Source: CAD feature listing. Evaluate the final solid. Frame: model axes, mm. Face numbers are marked on the shaded views. A direction names the side the tool comes from. Give positions to 0.01 mm unless a question says otherwise; leave off trailing zeros. Write each loop counter-clockwise with the first axis right and the second up, starting at its lowest first coordinate (ties: lowest second). Pieces come first, ordered by that corner, then holes. Notation, with made-up numbers: (38, -22.75) -> (95, -22.75) arc R32 ccw to (95, 15.25) -> close; hole circle Ø10 at (-31.5, -31.5). An arc over 180 degrees is marked (long way). Use a Markdown table: item, result. Add a question column.
```python
from build123d import *

# Parameters (mm, degrees)
SKETCH1_W           = 120
SKETCH1_H           = 25
BOSS_EXTRUDE4_DEPTH = 1
SKETCH6_W           = 76
SKETCH6_H           = 7.5
CUT_EXTRUDE1_DEPTH  = 62.296410988
SKETCH7_W           = 1
SKETCH7_H           = 25
BOSS_EXTRUDE5_DEPTH = 23
SKETCH11_R          = 1.5
SKETCH11_W          = 6
SKETCH11_H          = 12
CUT_EXTRUDE3_DEPTH  = 66.819829839
CUT_EXTRUDE4_DEPTH  = 1
CUT_EXTRUDE5_DEPTH  = 1
BOSS_EXTRUDE6_DEPTH = 1
SKETCH13_W          = 22
SKETCH13_H          = 1
BOSS_EXTRUDE7_DEPTH = 1
SKETCH16_R          = 1.5
CUT_EXTRUDE6_DEPTH  = 1
SKETCH17_R          = 1.5
CUT_EXTRUDE7_DEPTH  = 1
CUT_EXTRUDE8_REACH  = 69.218


with BuildPart() as part:
    # Sketch1 → Boss-Extrude4 (new body)
    with BuildSketch(Plane.XY):
        Rectangle(SKETCH1_W, SKETCH1_H)
    extrude(amount=BOSS_EXTRUDE4_DEPTH)

    # Sketch6 → Cut-Extrude1 (cut, through all)
    with BuildSketch(Plane(origin=(0, 0, 0), x_dir=(-1, 0, 0), z_dir=(0, 0, -1))):
        with Locations((0, 8.75)):
            Rectangle(SKETCH6_W, SKETCH6_H)
        with Locations((0, -8.75)):
            Rectangle(SKETCH6_W, SKETCH6_H)
    extrude(amount=-CUT_EXTRUDE1_DEPTH, mode=Mode.SUBTRACT)

    # Sketch7 → Boss-Extrude5 (add)
    with BuildSketch(Plane.XY.offset(1)):
        with Locations((-38.5, 0)):
            Rectangle(SKETCH7_W, SKETCH7_H)
    extrude(amount=BOSS_EXTRUDE5_DEPTH)

    # Sketch11 → Cut-Extrude3 (cut, through all)
    with BuildSketch(Plane(origin=(0, 0, 0), x_dir=(-1, 0, 0), z_dir=(0, 0, -1))):
        with Locations((-49, 10)):
            Circle(SKETCH11_R)
        with Locations((-49, -10)):
            Circle(SKETCH11_R)
        with Locations((-49, 0)):
            Rectangle(SKETCH11_W, SKETCH11_H)
    extrude(amount=-CUT_EXTRUDE3_DEPTH, mode=Mode.SUBTRACT)

    # Sketch14 → Cut-Extrude4 (cut)
    with BuildSketch(Plane(origin=(0, 12.5, 0), x_dir=(1, 0, 0), z_dir=(0, 1, 0))):
        Polygon((-60, -1), (-39, -1), (-39, -24), (-38, -24), (-38, 0), (-60, 0), align=None)
    extrude(amount=-CUT_EXTRUDE4_DEPTH, mode=Mode.SUBTRACT)

    # Sketch15 → Cut-Extrude5 (cut)
    with BuildSketch(Plane.XZ.offset(12.5)):
        Polygon((-60, 0), (-38, 0), (-38, 24), (-39, 24), (-39, 1), (-60, 1), align=None)
    extrude(amount=-CUT_EXTRUDE5_DEPTH, mode=Mode.SUBTRACT)

    # Sketch10 → Boss-Extrude6 (add)
    with BuildSketch(Plane(origin=(0, 5, 0), x_dir=(1, 0, 0), z_dir=(0, 1, 0))):
        Polygon((-38, -1), (-38, -24), (60, -1), align=None)
    boss_extrude6 = extrude(amount=-BOSS_EXTRUDE6_DEPTH)

    # Mirror1: Boss-Extrude6 across plane
    add(boss_extrude6.mirror(Plane(origin=(0, 0, 0), x_dir=(0, 0, 1), z_dir=(0, -1, 0))))

    # Sketch13 → Boss-Extrude7 (add)
    with BuildSketch(Plane(origin=(0, -12.5, 0), x_dir=(-1, 0, 0), z_dir=(0, -1, 0))):
        with Locations((-49, -0.5)):
            Rectangle(SKETCH13_W, SKETCH13_H)
    boss_extrude7 = extrude(amount=BOSS_EXTRUDE7_DEPTH)

    # Mirror2: Boss-Extrude7 across plane
    add(boss_extrude7.mirror(Plane(origin=(0, 0, 0), x_dir=(0, 0, 1), z_dir=(0, -1, 0))))

    # Sketch16 → Cut-Extrude6 (cut)
    with BuildSketch(Plane(origin=(-38, 0, 0), x_dir=(0, 0, -1), z_dir=(1, 0, 0))):
        with Locations(Location((-12, -8.25, 0), (0, 0, 90))):
            Circle(SKETCH16_R)
        with Locations(Location((-12, 8.25, 0), (0, 0, 90))):
            Circle(SKETCH16_R)
    extrude(amount=-CUT_EXTRUDE6_DEPTH, mode=Mode.SUBTRACT)

    # Sketch17 → Cut-Extrude7 (cut)
    with BuildSketch(Plane.XY.offset(1)):
        with Locations((-49.5, 0)):
            Circle(SKETCH17_R)
    extrude(amount=-CUT_EXTRUDE7_DEPTH, mode=Mode.SUBTRACT)

    # Cut-Extrude8: up to this face of the body (flat: up to its plane)
    cut_extrude8_end = Plane(part.part.faces().sort_by_distance((-4.996397894, -5, 8.150734275))[0])
    # Sketch18 → Cut-Extrude8 (cut, up to the picked face)
    with BuildSketch(Plane(origin=(0, 5, 0), x_dir=(1, 0, 0), z_dir=(0, 1, 0)), mode=Mode.PRIVATE) as cut_extrude8_sk1:
        Polygon((-35, -6.994072078), (-35, -20.214403976), (-23.128514946, -17.428239116), align=None)
    cut_extrude8_tool1 = split(extrude(cut_extrude8_sk1.sketch, amount=-CUT_EXTRUDE8_REACH, mode=Mode.PRIVATE), bisect_by=cut_extrude8_end, keep=Keep.BOTH, mode=Mode.PRIVATE)
    # Sketch18 → Cut-Extrude8 (cut, up to the picked face)
    with BuildSketch(Plane(origin=(0, 5, 0), x_dir=(1, 0, 0), z_dir=(0, 1, 0)), mode=Mode.PRIVATE) as cut_extrude8_sk2:
        Polygon((38.348329984, -3), (27.953371723, -3), (33.784828112, -4.071025949), align=None)
    cut_extrude8_tool2 = split(extrude(cut_extrude8_sk2.sketch, amount=-CUT_EXTRUDE8_REACH, mode=Mode.PRIVATE), bisect_by=cut_extrude8_end, keep=Keep.BOTH, mode=Mode.PRIVATE)
    # Sketch18 → Cut-Extrude8 (cut, up to the picked face)
    with BuildSketch(Plane(origin=(0, 5, 0), x_dir=(1, 0, 0), z_dir=(0, 1, 0)), mode=Mode.PRIVATE) as cut_extrude8_sk3:
        Polygon((-35, -3), (-22.366422742, -14.103990342), (-12.606827419, -3), align=None)
    cut_extrude8_tool3 = split(extrude(cut_extrude8_sk3.sketch, amount=-CUT_EXTRUDE8_REACH, mode=Mode.PRIVATE), bisect_by=cut_extrude8_end, keep=Keep.BOTH, mode=Mode.PRIVATE)
    # Sketch18 → Cut-Extrude8 (cut, up to the picked face)
    with BuildSketch(Plane(origin=(0, 5, 0), x_dir=(1, 0, 0), z_dir=(0, 1, 0)), mode=Mode.PRIVATE) as cut_extrude8_sk4:
        Polygon((-20.817385235, -16.885831123), (-9.723935411, -4.264246351), (14.222143926, -8.662268156), align=None)
    cut_extrude8_tool4 = split(extrude(cut_extrude8_sk4.sketch, amount=-CUT_EXTRUDE8_REACH, mode=Mode.PRIVATE), bisect_by=cut_extrude8_end, keep=Keep.BOTH, mode=Mode.PRIVATE)
    # Sketch18 → Cut-Extrude8 (cut, up to the picked face)
    with BuildSketch(Plane(origin=(0, 5, 0), x_dir=(1, 0, 0), z_dir=(0, 1, 0)), mode=Mode.PRIVATE) as cut_extrude8_sk5:
        Polygon((14.690257392, -5.69806474), (18.253543406, -3), (0, -3), align=None)
    cut_extrude8_tool5 = split(extrude(cut_extrude8_sk5.sketch, amount=-CUT_EXTRUDE8_REACH, mode=Mode.PRIVATE), bisect_by=cut_extrude8_end, keep=Keep.BOTH, mode=Mode.PRIVATE)
    # Sketch18 → Cut-Extrude8 (cut, up to the picked face)
    with BuildSketch(Plane(origin=(0, 5, 0), x_dir=(1, 0, 0), z_dir=(0, 1, 0)), mode=Mode.PRIVATE) as cut_extrude8_sk6:
        Polygon((20.904659834, -4.755587386), (26.493983886, -5.782142452), (16.429296354, -8.144262995), align=None)
    cut_extrude8_tool6 = split(extrude(cut_extrude8_sk6.sketch, amount=-CUT_EXTRUDE8_REACH, mode=Mode.PRIVATE), bisect_by=cut_extrude8_end, keep=Keep.BOTH, mode=Mode.PRIVATE)
    add(cut_extrude8_tool1.solids().sort_by(Axis((-31.042838, 5, 14.878905), (0, -1, 0)))[0], mode=Mode.SUBTRACT)
    add(cut_extrude8_tool2.solids().sort_by(Axis((33.362177, 5, 3.357009), (0, -1, 0)))[0], mode=Mode.SUBTRACT)
    add(cut_extrude8_tool3.solids().sort_by(Axis((-23.324417, 5, 6.70133), (0, -1, 0)))[0], mode=Mode.SUBTRACT)
    add(cut_extrude8_tool4.solids().sort_by(Axis((-5.439726, 5, 9.937449), (0, -1, 0)))[0], mode=Mode.SUBTRACT)
    add(cut_extrude8_tool5.solids().sort_by(Axis((10.981267, 5, 3.899355), (0, -1, 0)))[0], mode=Mode.SUBTRACT)
    add(cut_extrude8_tool6.solids().sort_by(Axis((21.27598, 5, 6.227331), (0, -1, 0)))[0], mode=Mode.SUBTRACT)


solid = part.part
```
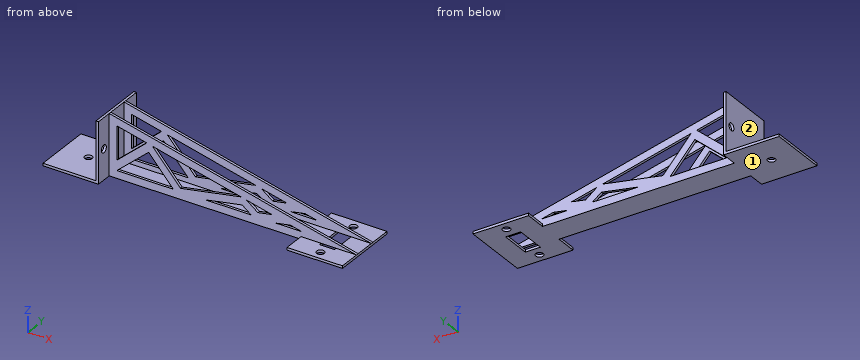
(1) Material intervals for L1, parallel to Y at x = 49, z = 0.3; L2, parallel to Z at x = -38.3, y = 8.25; L3, parallel to Y at x = -49.5, z = 0.75, sorted ascending.
(2) Cut plane C-C on z = 22.5. Return the cut outline in (x, y).
(3) Cut plane D-D on z = 12. Count the separate pieces of the cut face and the enclosed holes in it, then the cut area to 3 significant figures.
(4) First-contact query: pin 1 Ø5 at (y, z) = (-8.5, 15) entering from +X; pin 2 Ø1.1 at (x, y) = (-23.5, -4.5) entering from +Z; pin 3 Ø2.5 at (x, y) = (47, 9) entering from +Z. Flat tips, straight axial feed; report the tip coordinate or a pass-through.
(5) Cut plane B-B on x = 6. Return the cut outline in (y, z).
(6) Cut plane A-A on y = -2.75. Return the cut outline in (x, z).
(7) Access query for the marked faces 1 and 2. Directions: +Z, -Z, +X, -X, +Y, -Y. A direction counts if a zero-diameter tool reaches every point of the face in a straight line with its end or side. Return the directions, or none.
Output:
| question | item | result |
|---|---|---|
| 1 | L1 | -13.5 to -11.5, -8.5 to -6, 6 to 8.5, 11.5 to 13.5 |
| 1 | L2 | 0 to 10.5, 13.5 to 24 |
| 1 | L3 | -11.5 to -1.5, 1.5 to 11.5 |
| 2 | outline | (-39, -11.5) -> (-38, -11.5) -> (-38, -5) -> (-31.61, -5) -> (-31.61, -4) -> (-38, -4) -> (-38, 4) -> (-31.61, 4) -> (-31.61, 5) -> (-38, 5) -> (-38, 11.5) -> (-39, 11.5) -> close |
| 3 | separate pieces | 9 |
| 3 | enclosed holes | 0 |
| 3 | area | 66.3 mm^2 |
| 4 | pin 1 | x = -38 |
| 4 | pin 2 | z = 20.73 |
| 4 | pin 3 | z = 1 |
| 5 | outline | (-5, 0) -> (5, 0) -> (5, 3) -> (4, 3) -> (4, 1) -> (-4, 1) -> (-4, 3) -> (-5, 3) -> close; (-5, 4.1) -> (-4, 4.1) -> (-4, 7.15) -> (-5, 7.15) -> close; (-5, 10.59) -> (-4, 10.59) -> (-4, 13.67) -> (-5, 13.67) -> close; (4, 4.1) -> (5, 4.1) -> (5, 7.15) -> (4, 7.15) -> close; (4, 10.59) -> (5, 10.59) -> (5, 13.67) -> (4, 13.67) -> close |
| 6 | outline | (-60, 0) -> (46, 0) -> (46, 1) -> (-38, 1) -> (-38, 24) -> (-39, 24) -> (-39, 1) -> (-60, 1) -> close; (52, 0) -> (60, 0) -> (60, 1) -> (52, 1) -> close |
| 7 | face 1 | -Z, +X, -X, +Y, -Y |
| 7 | face 2 | +Z, -X, +Y, -Y |
